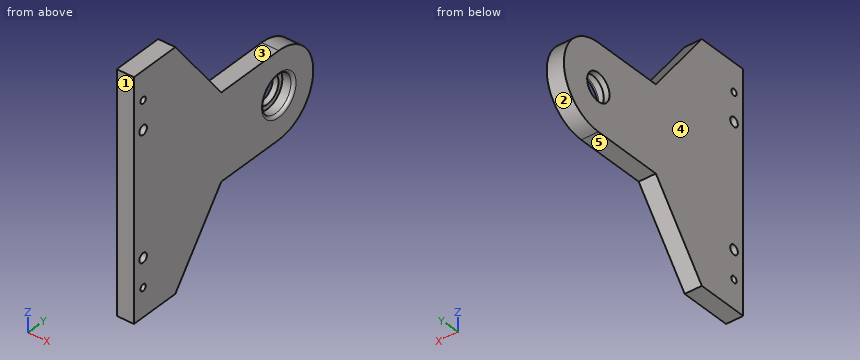
Autodesk Inventor part; units mm, degrees
ref_plane "YZ Plane" through (0, 0, 0) normal (1, 0, 0) x (0, 1, 0)
ref_plane "XZ Plane" through (0, 0, 0) normal (0, 1, 0) x (-1, 0, 0)
ref_plane "XY Plane" through (0, 0, 0) normal (0, 0, 1) x (1, 0, 0)
sketch "스케치1" plane through (0, 0, 0) normal (1, 0, 0) x (0, 1, 0)
  line L0 (0, -41.5) -> (18, -41.5)
  line L1 (18, -41.5) -> (18, 59.6584) construction
  line L2 (0, 0) -> (0, -41.5)
  line L3 (84.3904, 0) -> (-15.1692, 0) construction
  arc A0 (63, -15) -> (78, 0) centre (63, 0) ccw
  line L4 (63, -15) -> (38, -15)
  line L5 (38, -15) -> (18, -41.5)
  line L6 (0, 41.5) -> (18, 41.5)
  line L7 (0, 0) -> (0, 41.5)
  arc A1 (78, 0) -> (63, 15) centre (63, 0) ccw
  line L8 (63, 15) -> (38, 15)
  line L9 (38, 15) -> (18, 41.5)
  dimension "d0" = 18
  dimension "d8" = 45
  dimension "d9" = 25
extrude "돌출1" add sketch "스케치1" along normal blind 6
sketch "스케치2" plane through (6, 0, 0) normal (1, 0, 0) x (0, 0, -1)
  line L0 (-58.8675, 4) -> (65.7315, 4) construction
  line L1 (-41.5, 0) -> (41.5, 0)
  circle A0 centre (31.5, 4) radius 1.15
  circle A1 centre (21.5, 4) radius 1.65
  line L2 (41.5, 0) -> (41.5, 18)
  line L3 (0, 13.8041) -> (0, -7.7982) construction
  circle A2 centre (-31.5, 4) radius 1.15
  circle A3 centre (-21.5, 4) radius 1.65
  point P0 (0, 0)
  dimension "d12" = 4
  dimension "d13" = 2.3
  dimension "d14" = 3.3
  dimension "d15" = 10
  dimension "d16" = 20
extrude "돌출2" cut sketch "스케치2" against normal blind 6
sketch "스케치4" plane through (6, 0, 0) normal (1, 0, 0) x (0, 0, -1)
  arc A0 (15, 63) -> (-15, 63) centre (0, 63) ccw
  circle A1 centre (0, 63) radius 6.5
  point P0 (0, 0)
  dimension "d25" = 13
extrude "돌출4" cut sketch "스케치4" against normal blind 4
sketch "스케치5" plane through (2, 63, 0) normal (1, 0, 0) x (0, 0, -1)
  circle A0 centre (0, 0) radius 4.85
  point P0 (0, -63)
  dimension "d28" = 9.7
extrude "돌출5" cut sketch "스케치5" against normal blind 2
fillet "모깎기1" radius 1 1 edges at (6, 63, 6.5)
properties part number "탑(옆면수정)"
Part model, mm, in its own coordinate system. Face numbers are marked on the shaded views. A direction names the side the tool comes from. Round coordinates to 2 decimals unless told otherwise and drop trailing zeros. Loops run counter-clockwise (first coordinate to the right, second up) from the corner with the lowest first, then second, coordinate; pieces in that order, holes last.
1. Slice it at A-A (x = 4). Give the cut face in (y, z).
Solutions:
outline: (0, -41.5) - (18, -41.5) - (38, -15) - (63, -15) arc R15 ccw to (63, 15) - (38, 15) - (18, 41.5) - (0, 41.5) - close; hole circle Ø3.3 at (4, -21.5); hole circle Ø3.3 at (4, 21.5); hole circle Ø2.3 at (4, -31.5); hole circle Ø2.3 at (4, 31.5); hole circle Ø13 at (63, 0)
2. Slice it at B-B (z = 31.5). Give the cut face in (x, y), and give its area (3 significant figures).
Solutions:
outline: (0, 0) - (6, 0) - (6, 2.85) - (0, 2.85) - close; (0, 5.15) - (6, 5.15) - (6, 25.55) - (0, 25.55) - close
area: 139 mm2
3. Drill centre lines: line 1 along Y through (x, z) = (1.6, 0); line 2 along Y through (x, z) = (3.95, 0); line 3 along X through (y, z) = (66.5, 5). Where is each one in solid material? Low to high.
Solutions:
line 1: y = 0 to 58.15, 67.85 to 78
line 2: y = 0 to 56.5, 69.5 to 78
line 3: x = 0 to 2
4. Slice it at C-C (y = 39). Give the cut face in (x, z).
Solutions:
outline: (0, -15) - (6, -15) - (6, 15) - (0, 15) - close
5. Slice it at D-D (z = -11). Give the cut face in (x, y).
Solutions:
outline: (0, 0) - (6, 0) - (6, 73.2) - (0, 73.2) - close
6. 3-axis set-ups, long thin cutter, end or side, ignore diameter. For the marked faces 4 and 5: which of +Z, -Z, +X, -X, +Y, -Y reach the whole face in a straight line?
Solutions:
face 4: +Z, -Z, -X, +Y, -Y
face 5: -Z, +X, -X, +Y
7. Flat gauge pins, fed straight in: pin 1 (3 mm diameter, centred on x = 2, y = 33.5, fed in from +Z); pin 2 (1.5 mm diameter, centred on x = 5, z = -1, fed in from +Y); pin 3 (3 mm diameter, centred on x = 2, y = 52, fed in from -Z). Where does each tip first touch, or does it go through?
Solutions:
pin 1: stops at z = 22.95
pin 2: stops at y = 78
pin 3: stops at z = -15
8. Two-plate mould, pull along Y, no slides. Class the marked faces 1, 2 and 3: pulls with the +Y half, pulls with the -Y half, needs draft (parallel to the pull), parting line crosses it, or undercut.
Solutions:
face 1: pulls with the -Y half
face 2: pulls with the +Y half
face 3: needs draft
